Build history of the part. All positions in model axes, mm. A direction names the side the tool comes from. Round coordinates to 2 decimals unless told otherwise and drop trailing zeros. Order: outer loops, then holes, each group sorted by start corner. A loop starts at its lowest first (then second) coordinate and runs counter-clockwise, first axis right, second up. Notation, with made-up numbers: (-39, -21.75) -> (-25, -21.75) arc R20 cw to (-25, -14.75) -> close; hole circle Ø5 at (86.5, 58). An arc over 180 degrees is marked (long way). Answer as CSV lines item,"result". Start each with the question number.
```python
from build123d import *

# Parameters (mm, degrees)
SCHIZZO1_R                   = 7
ESTRUSIONE_ESTRUSIONE1_DEPTH = 100
TAGLIO_ESTRUSIONE1_REACH     = 202.245
SCHIZZO2_R                   = 2
SCHIZZO5_R                   = 4.87
TAGLIO_ESTRUSIONE2_DEPTH     = 4
FORO_PER_VITE_M8_1_D         = 8.4
FORO_PER_VITE_M8_1_DEPTH     = 2
FORO_PER_VITE_M8_1_TIP       = 2.5236146


with BuildPart() as part:
    # Schizzo1 → Estrusione-Estrusione1 (new, symmetric)
    with BuildSketch(Plane.XY):
        Circle(SCHIZZO1_R)
    extrude(amount=ESTRUSIONE_ESTRUSIONE1_DEPTH, both=True)

    # Schizzo2 → Taglio-Estrusione1 (cut, up to next)
    with BuildSketch(Plane.XY.offset(100), mode=Mode.PRIVATE) as taglio_estrusione1_sk1:
        Circle(SCHIZZO2_R)
    taglio_estrusione1_tool1 = extrude(taglio_estrusione1_sk1.sketch, amount=-TAGLIO_ESTRUSIONE1_REACH, mode=Mode.PRIVATE) & part.part
    add(taglio_estrusione1_tool1.solids().sort_by_distance((0, 0, 100))[0], mode=Mode.SUBTRACT)

    # Schizzo5 → Taglio-Estrusione2 (cut)
    with BuildSketch(Plane.XY.offset(100)):
        Circle(SCHIZZO5_R)
    extrude(amount=-TAGLIO_ESTRUSIONE2_DEPTH, mode=Mode.SUBTRACT)

    # Foro per Vite M8-1
    with Locations(Plane(origin=(7, 0, 0), x_dir=(0, 0, -1), z_dir=(1, 0, 0))):
        with Locations((0, 0)):
            Hole(FORO_PER_VITE_M8_1_D / 2, depth=FORO_PER_VITE_M8_1_DEPTH)
            with Locations((0, 0, -(FORO_PER_VITE_M8_1_DEPTH + FORO_PER_VITE_M8_1_TIP / 2))):  # 118° drill point
                Cone(0, FORO_PER_VITE_M8_1_D / 2, FORO_PER_VITE_M8_1_TIP, mode=Mode.SUBTRACT)


solid = part.part
```
Q1. Which spindle directions (+Z, -Z, +X, -X, +Y, -Y) get a long thin tool onto all of the face, cutting with end or side? Do faces 1 (the face through (1, -2, 96)), 2 (the face through (2.915, 0.219, -0.696)). Say none if no direction does.
Q2. Flat gauge pins, fed straight in: pin 1 Ø5 at (y, z) = (3.5, -11) entering from -X; pin 2 Ø8 at (y, z) = (5.5, 52) entering from +X; pin 3 Ø6.5 at (y, z) = (0, 0) entering from +X; pin 4 Ø2.5 at (x, y) = (0, 0) entering from -Z. Where does each tip first touch, or does it go through?
Q3. Two-plate mould, pull along Z, no slides. Class faces 3 (the face through (1, 5, 100)), 4 (the face through (5.76, 3.54, 2.26)), 5 (the face through (0, -2, -1)): +Z half, -Z half, draft (parallel to the pull), parting line (faces both ways), or undercut.
Q4. Probe L1, parallel to X at y = 0.25, z = -84; L2, parallel to Z at x = 5.55, y = 0; L3, parallel to Z at x = 1.75, y = -2.5. List the from-to ranges inside material, lowest first.
Q5. Slice it at B-B, the plane z = 60. Write the cut outline in (x, y), plus the area to 3 significant figures.
Q6. Slice it at A-A, the plane x = 0. Write the cut outline in (y, z).
Solutions:
1,face 1,"+Z"
1,face 2,"+X"
2,pin 1,"stops at x = -6.93"
2,pin 2,"stops at x = 6.84"
2,pin 3,"stops at x = 4.43"
2,pin 4,"passes through"
3,face 3,"+Z half"
3,face 4,"undercut"
3,face 5,"draft"
4,L1,"x = -7 to -1.98, 1.98 to 7"
4,L2,"z = -100 to -4.2, 4.2 to 100"
4,L3,"z = -100 to 96"
5,outline,"circle Ø14 at (0, 0); hole circle Ø4 at (0, 0)"
5,area,"141 mm2"
6,outline,"(-7, -100) -> (-2, -100) -> (-2, 96) -> (-4.87, 96) -> (-4.87, 100) -> (-7, 100) -> close; (2, -100) -> (7, -100) -> (7, 100) -> (4.87, 100) -> (4.87, 96) -> (2, 96) -> close"
